Here's how the part is built. I have some questions about the finished solid (model axes, mm). A direction names the side the tool comes from. Coordinates: 2 decimals unless noted, no trailing zeros. Write each loop counter-clockwise with the first axis right and the second up, starting at its lowest first coordinate (ties: lowest second). Pieces come first, ordered by that corner, then holes. Notation, with made-up numbers: (62.5, -19) - (75.5, -19) arc R19 ccw to (75.5, -8) - close; hole circle Ø7 at (59.5, 13.5). An arc over 180 degrees is marked (long way). Answer in a Markdown table with one row per item. Add a question column.
Item 1: Imagine slicing it at A-A (z = 14.5). Please give me the cut outline in (x, y), plus the area to 3 significant figures.
Item 2: Imagine slicing it at B-B (x = 173.5). Please give me the cut outline in (y, z), plus the area to 3 significant figures.
Item 3: I'm going to push flat-ended pins straight in: pin 1 (4 mm diameter, centred on y = -28.5, z = -83, fed in from -X); pin 2 (1 mm diameter, centred on x = -323.5, y = -5.5, fed in from -Z). Where does each tip first touch, or does it pass through?
Item 4: If I drill on probe 1 along Y at (x, z) = (245.5, 124); probe 2 along Z at (x, y) = (246.25, 60); probe 3 along X at (y, z) = (6.5, -133), over which ranges is the centre line in solid material (lowest first)? Write a range as from..to.
Item 5: Which directions (+Z, -Z, +X, -X, +Y, -Y) give clear straight access to the entire face, cutting with the end or side of a thin tool? Please do faces 1 (the face through (254, 1, -78)), 2 (the face through (-206.586, 15.569, -29.097)).
Autodesk Inventor part; units mm, degrees
ref_plane "YZ Plane" through (0, 0, 0) normal (1, 0, 0) x (0, 1, 0)
ref_plane "XZ Plane" through (0, 0, 0) normal (0, 1, 0) x (-1, 0, 0)
ref_plane "XY Plane" through (0, 0, 0) normal (0, 0, 1) x (1, 0, 0)
sketch "Sketch1" plane through (0, 0, 0) normal (1, 0, 0) x (0, 1, 0)
  circle A0 centre (0, 0) radius 33
extrude "Extrusion1" add sketch "Sketch1" against normal blind 600
sketch "Sketch2" plane through (0, 0, 0) normal (1, 0, 0) x (0, 0, -1)
  circle A0 centre (0, 0) radius 33
extrude "Extrusion2" add sketch "Sketch2" along normal blind 198
sketch "Sketch3" plane through (198, 0, 0) normal (1, 0, 0) x (0, 0, -1)
  circle A0 centre (0, 0) radius 103
extrude "Extrusion3" add sketch "Sketch3" along normal blind 36
sketch "Sketch4" plane through (234, 0, 0) normal (1, 0, 0) x (0, 0, -1)
  line L0 (-212, 107) -> (212, 107)
  line L1 (212, -107) -> (-212, -107)
  line L2 (-212, -107) -> (-212, 107)
  line L3 (-212, 107) -> (212, -107) construction
  line L4 (212, 107) -> (-212, -107) construction
  line L5 (212, 107) -> (376, 107)
  line L6 (376, 107) -> (376, -107)
  line L7 (376, -107) -> (212, -107)
  point P0 (0, 0)
  point P1 (0, 0)
extrude "Extrusion4" add sketch "Sketch4" along normal blind 20
sketch "Sketch5" plane through (254, 0, 0) normal (1, 0, 0) x (0, 0, -1)
  point P0 (0, 0)
  point P1 (-124.0692, -60)
  point P2 (-124, 60)
  point P3 (220, 60)
  point P4 (220, -60)
hole "Hole1" at (254, -60, 124.0692) at (254, 60, 124) at (254, 60, -220) at (254, -60, -220) direction (-1, 0, 0) diameter 6.647 depth 20
properties part number "DecAxis"
Here are the results:
| question | item | result |
|---|---|---|
| 1 | outline | (-600, -29.64) - (198, -29.64) - (198, -101.97) - (234, -101.97) - (234, -107) - (254, -107) - (254, 107) - (234, 107) - (234, 101.97) - (198, 101.97) - (198, 29.64) - (-600, 29.64) - close |
| 1 | area | 58,900 mm2 |
| 2 | outline | circle Ø66 at (0, 0) |
| 2 | area | 3,420 mm2 |
| 3 | pin 1 | stops at x = 198 |
| 3 | pin 2 | stops at z = -32.62 |
| 4 | probe 1 | y = -107..-63.32, -56.68..56.68, 63.32..107 |
| 4 | probe 2 | z = -376..-223.32, -216.68..120.68, 127.32..212 |
| 4 | probe 3 | x = 234..254 |
| 5 | face 1 | +Z, -Z, +X, +Y, -Y |
| 5 | face 2 | -X |
